Answer from the drawing. Dimensions are ordinates in mm from the lowest x, y and z of the part. A direction names the side the tool comes from. Round coordinates to 2 decimals unless told otherwise and drop trailing zeros. Write each loop counter-clockwise with the first axis right and the second up, starting at its lowest first coordinate (ties: lowest second). Pieces come first, ordered by that corner, then holes. Notation, with made-up numbers: (83.25, -30) -> (113.25, -30) arc R25 ccw to (113.25, -5) -> close; hole circle Ø6 at (-25, 14.25). An arc over 180 degrees is marked (long way). Return JSON: item names as keys, results as strings. Group by question number.
(1) A cutting plane is placed at C-C on x = 47.5. Give the vertices of the cut face in (y, z), then the cut area to 3 significant figures.
(2) A cutting plane is placed at B-B on y = 33.5. Give the vertices of the cut face in (x, z).
(3) A cutting plane is placed at A-A on y = 24. Give the vertices of the cut face in (x, z).
(4) A cutting plane is placed at D-D on y = 8.5. Give the vertices of the cut face in (x, z), then the cut area to 3 significant figures.
(5) For the marked faces 1, 2 and 3, determine the directions among +Z, -Z, +X, -X, +Y, -Y from which every point of the face is accessible in a straight line to the end or side of a thin tool.
(6) The mould has two halves that part along Z. Classify the marked faces 4, 5 and 6: released by +Z, released by -Z, zero draft, split by the parting line, or undercut.
(7) Straight lines are drawn through the part: line 1 (Z direction, x = 44, y = 24.25); line 2 (Z direction, x = 37, y = 26) (3 decimals); line 3 (Z direction, x = 44, y = 33.75). For each, find the intervals that lie inside material, in ascending order.
(8) Given pin 1 (20 mm diameter, centred on x = 41.5, z = 71, fed in from -Y); pin 2 (4 mm diameter, centred on x = 68.5, y = 27.5, fed in from +Z); pin 3 (5 mm diameter, centred on y = 31.5, z = 82, fed in from +X), each flat-ended and moving along its own axis, determine where each tip first touches the part or whether it passes through.
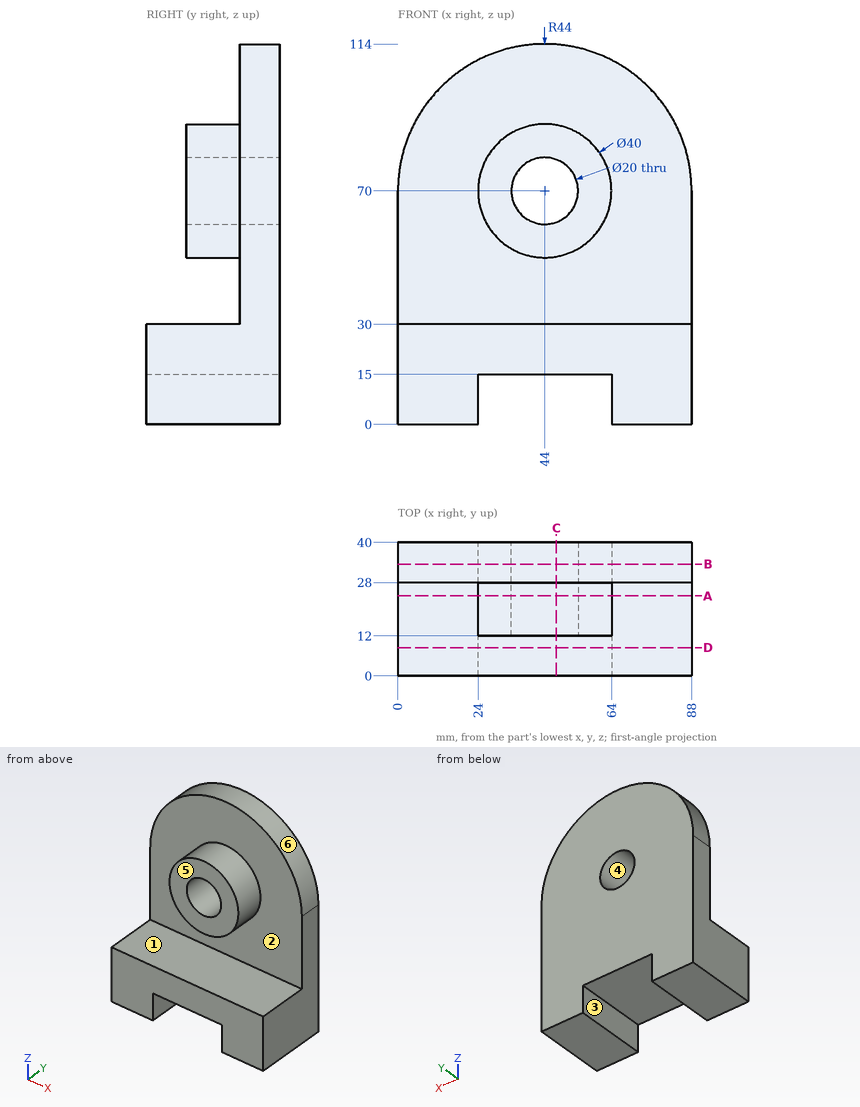
Checks:
{
 "1": {"outline": "(0, 15) -> (40, 15) -> (40, 60.63) -> (12, 60.63) -> (12, 50.31) -> (28, 50.31) -> (28, 30) -> (0, 30) -> close; (12, 79.37) -> (40, 79.37) -> (40, 113.86) -> (28, 113.86) -> (28, 89.69) -> (12, 89.69) -> close", "area": "1,710 mm^2"},
 "2": {"outline": "(0, 0) -> (24, 0) -> (24, 15) -> (64, 15) -> (64, 0) -> (88, 0) -> (88, 70) arc R44 ccw to (0, 70) -> close; hole circle Ø20 at (44, 70)"},
 "3": {"outline": "(0, 0) -> (24, 0) -> (24, 15) -> (64, 15) -> (64, 0) -> (88, 0) -> (88, 30) -> (0, 30) -> close; circle Ø40 at (44, 70); hole circle Ø20 at (44, 70)"},
 "4": {"outline": "(0, 0) -> (24, 0) -> (24, 15) -> (64, 15) -> (64, 0) -> (88, 0) -> (88, 30) -> (0, 30) -> close", "area": "2,040 mm^2"},
 "5": {"face 1": "+X, -X, -Y", "face 2": "-Y", "face 3": "-Z, +Y, -Y"},
 "6": {"face 4": "undercut", "face 5": "zero draft", "face 6": "released by +Z"},
 "7": {"line 1": "z = 15 to 30, 50 to 60, 80 to 90", "line 2": "z = 15 to 30, 51.265 to 62.859, 77.141 to 88.735", "line 3": "z = 15 to 60, 80 to 114"},
 "8": {"pin 1": "stops at y = 12", "pin 2": "stops at z = 107.77", "pin 3": "stops at x = 86.96"}
}
